Input: part model. Units: mm. Frame: model coordinates. A direction names the side the tool comes from. Give positions to 0.01 mm unless a question says otherwise; leave off trailing zeros. Write each loop counter-clockwise with the first axis right and the second up, starting at its lowest first coordinate (ties: lowest second). Pieces come first, ordered by that corner, then holes. Notation, with made-up numbers: (42.5, 87.25) -> (96.5, 87.25) arc R13 cw to (96.5, 104.25) -> close; hole circle Ø4 at (53.25, -37.5). An arc over 180 degrees is marked (long way). Answer as a JSON object with one key per item and string values. Group by question number.
from build123d import *

# Parameters (mm, degrees)
F1_DEPTH      = 15
F3_DEPTH      = 200
F4_R          = 4.5
F5_DEPTH      = 25
F6_R          = 2
F8_DEPTH      = 30
F8_DEPTH_BACK = 30
F9_R          = 3.25
F10_DEPTH     = 25
F13_DEPTH     = 12
F14_R         = 3.25
F15_DEPTH     = 25
F16_R         = 2
F17_R         = 5


with BuildPart() as f1:
    # F0 (on Top) → F1 (new body)
    with BuildSketch(Plane.XY):
        Polygon((-10, -20), (10, -20), (10, 20), (5, 20), (5, -13), (-5, -13), (-5, 20), (-10, 20), align=None)
    extrude(amount=F1_DEPTH)

    # F2 (on face) → F3 (join)
    with BuildSketch(Plane.XZ.offset(20)):
        with BuildLine():
            ThreePointArc((0, 3), (3.1819805153, 4.3180194847), (4.5, 7.5))
            ThreePointArc((4.5, 7.5), (-3.1819805153, 10.6819805153), (0, 3))
        make_face()
    extrude(amount=F3_DEPTH)

    # F4 (on face) → F5 (cut)
    with BuildSketch(Plane(origin=(-10, 0, 0), x_dir=(0, -1, 0), z_dir=(-1, 0, 0))):
        with Locations((-13, 7.5)):
            Circle(F4_R)
    extrude(amount=-F5_DEPTH, mode=Mode.SUBTRACT)

    # F6
    f6_edges = [f1.edges().sort_by_distance(p)[0] for p in [
        (-7.5, 20, 15),
        (7.5, 20, 15),
        (7.5, 20, 0),
        (-7.5, 20, 0),
    ]]
    fillet(f6_edges, radius=F6_R)

    # F7 (on Right) → F8 (join, two sides)
    with BuildSketch(Plane.YZ) as f8_sk:
        Polygon((-210, -10.3205080757), (-220, 7), (-222.8867513459, 12), (-240, 41.6410161514), (-243.4641016151, 39.6410161514), (-213.4641016151, -12.3205080757), align=None)
        Polygon((-222.8867513459, 12), (-220, 7), (-220, 12), align=None)
    extrude(amount=F8_DEPTH)
    extrude(f8_sk.sketch, amount=-F8_DEPTH_BACK)

    # F9 (on face) → F10 (cut)
    with BuildSketch(Plane(origin=(0, -165.4330127019, -95.5127944163), x_dir=(1, 0, 0), z_dir=(0, -0.8660254038, -0.5))):
        with Locations((-22.5, 148.5621778265)):
            Circle(F9_R)
        with Locations((22.5, 148.5621778265)):
            Circle(F9_R)
        with Locations((-22.5, 103.5621778265)):
            Circle(F9_R)
        with Locations((22.5, 103.5621778265)):
            Circle(F9_R)
    extrude(amount=-F10_DEPTH, mode=Mode.SUBTRACT)

    # F12 (on offset) → F13 (join)
    with BuildSketch(Plane.XZ.offset(80)):
        with BuildLine():
            Line((-5, 0), (-5, -15))
            Line((-5, -15), (5, -15))
            Line((5, -15), (5, 0))
            Line((5, 0), (8.5, 0))
            Line((8.5, 0), (8.5, 10))
            Line((8.5, 10), (4.5, 10))
            Line((4.5, 10), (4.5, 7.5))
            ThreePointArc((4.5, 7.5), (0, 3), (-4.5, 7.5))
            Line((-4.5, 7.5), (-4.5, 10))
            Line((-4.5, 10), (-8.5, 10))
            Line((-8.5, 10), (-8.5, 0))
            Line((-8.5, 0), (-5, 0))
        make_face()
    extrude(amount=F13_DEPTH)

    # F14 (on face) → F15 (cut)
    with BuildSketch(Plane(origin=(-5, 0, 0), x_dir=(0, -1, 0), z_dir=(-1, 0, 0))):
        with Locations((86, -9)):
            Circle(F14_R)
    extrude(amount=-F15_DEPTH, mode=Mode.SUBTRACT)

    # F16
    f16_edges = [f1.edges().sort_by_distance(p)[0] for p in [
        (0, -80, -15),
        (0, -92, -15),
    ]]
    fillet(f16_edges, radius=F16_R)

    # F17
    f17_edges = [f1.edges().sort_by_distance(p)[0] for p in [
        (-30, -241.732051, 40.641016),
        (30, -241.732051, 40.641016),
        (-30, -211.732051, -11.320508),
        (30, -211.732051, -11.320508),
    ]]
    fillet(f17_edges, radius=F17_R)


solid = f1.part
1. Section D-D (y = -23). Return the cut outline in (x, z).
2. Reachability of faces 1 (the face through (0, -92, -1)), 2 (the face through (-7, -5, 15)), 3 (the face through (0, -13, 7)), 4 (the face through (-8.5, -86, 5)) from +Z, -Z, +X, -X, +Y, -Y: full face, straight path, thin tool, end or side. Return the list, or none.
3. Section A-A (y = 13). Return the cut outline in (x, z).
4. Mould query, pull axis Z, two halves, no side actions, for faces 5 (the face through (28.6, -212.5, -10)), 6 (the face through (21.8, -213.92, -7.59)), 7 (the face through (30, -227, 15)). Classes: pulls with the +Z half, pulls with the -Z half, needs draft (parallel to the pull), parting line crosses it, or undercut.
5. Section C-C (x = -15). Return the cut outline in (y, z).
6. Contact query for flat-ended pins moving along their axis: pin 1 Ø2 at (y, z) = (-85.5, 9) entering from -X; pin 2 Ø10 at (x, y) = (-3.5, -132) entering from +Z; pin 3 Ø3.5 at (y, z) = (-87, -10.5) entering from +X. Output: stop coordinate, or through.
7. Section B-B (y = -86). Return the cut outline in (x, z).
8. Line query: line 1 (Z direction, x = -8.05, y = 13); line 2 (Y direction, x = -7, z = 7); line 3 (Z direction, x = 2.25, y = -86). Output: solid intervals per line, ascending.
Working result:
{
 "1": {"outline": "circle Ø9 at (0, 7.5)"},
 "2": {"face 1": "-Z", "face 2": "+Z, +X, -X, +Y", "face 3": "+Z, -Z, +Y", "face 4": "+Z, -Z, -X"},
 "3": {"outline": "(-10, 0) -> (-5, 0) -> (-5, 3) -> (-10, 3) -> close; (-10, 12) -> (-5, 12) -> (-5, 15) -> (-10, 15) -> close; (5, 0) -> (10, 0) -> (10, 3) -> (5, 3) -> close; (5, 12) -> (10, 12) -> (10, 15) -> (5, 15) -> close"},
 "4": {"face 5": "pulls with the -Z half", "face 6": "undercut", "face 7": "needs draft"},
 "5": {"outline": "(-243.46, 39.64) -> (-213.46, -12.32) -> (-210, -10.32) -> (-220, 7) -> (-220, 12) -> (-222.89, 12) -> (-240, 41.64) -> close"},
 "6": {"pin 1": "stops at x = -8.5", "pin 2": "stops at z = 12", "pin 3": "stops at x = 5"},
 "7": {"outline": "(-8.5, 0) -> (-5, 0) -> (-5, -5.75) -> (5, -5.75) -> (5, 0) -> (8.5, 0) -> (8.5, 10) -> (4.5, 10) -> (4.5, 7.5) arc R4.5 ccw to (-4.5, 7.5) -> (-4.5, 10) -> (-8.5, 10) -> close; (-5, -15) -> (5, -15) -> (5, -12.25) -> (-5, -12.25) -> close"},
 "8": {"line 1": "z = 0 to 3, 12 to 15", "line 2": "y = -224.62 to -220, -92 to -80, -20 to 8.53, 17.47 to 20", "line 3": "z = -15 to -12.25, -5.75 to 11.4"}
}
